Verification items for this drawing (mm, ordinates from the low corner). A direction names the side the tool comes from. Round coordinates to 2 decimals unless told otherwise and drop trailing zeros. Loops run counter-clockwise (first coordinate to the right, second up) from the corner with the lowest first, then second, coordinate; pieces in that order, holes last. Notation, with made-up numbers: M 35.25,-14.5 L 77.25,-14.5 A24 cw 77.25,-2.5 Z; hole C 79.25,-14.5 d6. An arc over 180 degrees is marked long. Write item = value, one per line. Start each with the question number.
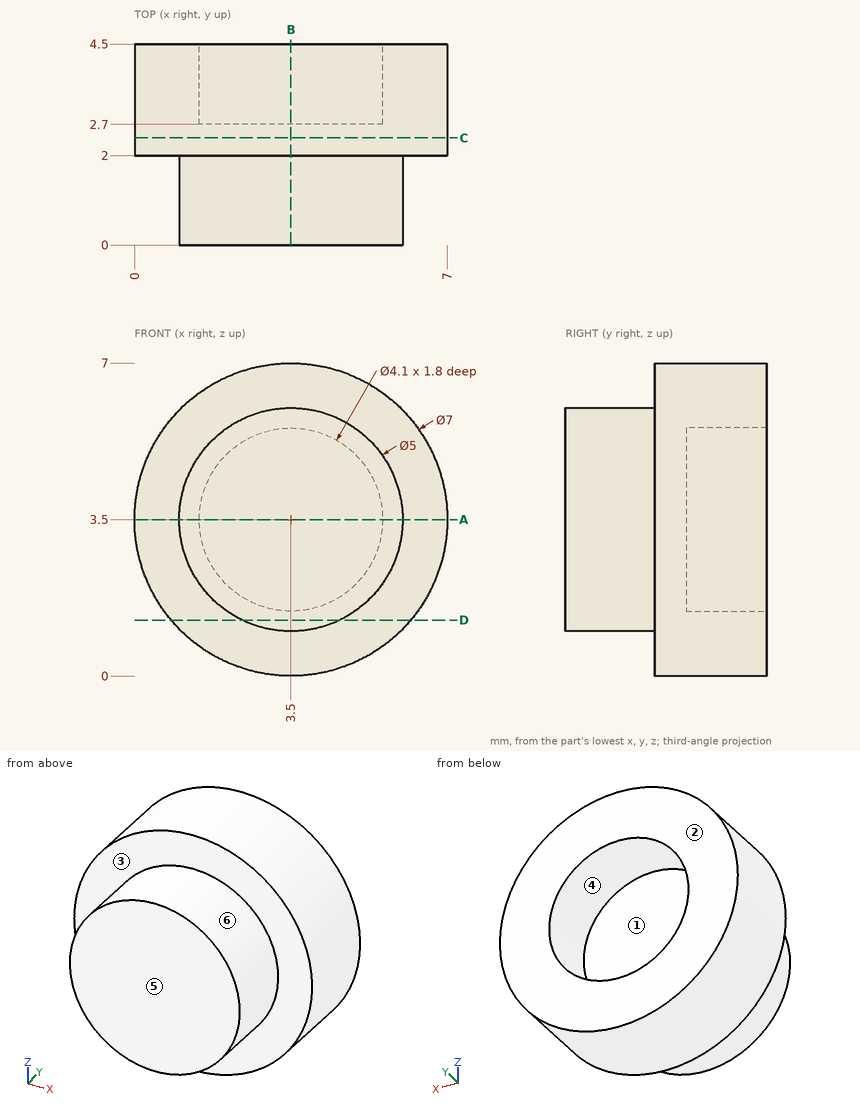
1. Section check D-D, the plane z = 1.25. Enter the section's corners in (x, y), and give its area (3 significant figures).
2. Section check C-C, the plane y = 2.4. Enter the section's corners in (x, z), and give its area (3 significant figures).
3. Thickness scan on line 1 (X direction, y = 3.7, z = 3.5); line 2 (Z direction, x = 4.5, y = 3.3); line 3 (Y direction, x = 6.5, z = 4.25). Record the ranges inside material, lowest first.
4. Tool access check on the marked faces 1, 2 and 3. Record the directions out of +Z, -Z, +X, -X, +Y, -Y that give a thin tool (end or side, any length) a straight path to the whole face; none if there is none.
5. Mould release check, pull along X, two halves, no side actions. Record for the marked faces 4, 5 and 6: pulls with the +X half, pulls with the -X half, needs draft (parallel to the pull), parting line crosses it, or undercut.
6. Section check B-B, the plane x = 3.5. Enter the section's corners in (y, z).
7. Section check A-A, the plane z = 3.5. Enter the section's corners in (x, y), and give its area (3 significant figures).
Computed values:
q1.outline = M 0.82,2 L 2.41,2 L 2.41,0 L 4.59,0 L 4.59,2 L 6.18,2 L 6.18,4.5 L 0.82,4.5 Z
q1.area = 17.8 mm2
q2.outline = C 3.5,3.5 d7
q2.area = 38.5 mm2
q3.line_1 = 0 to 1.45, 5.55 to 7
q3.line_2 = 0.15 to 1.71, 5.29 to 6.85
q3.line_3 = 2 to 4.5
q4.face_1 = +Y
q4.face_2 = +Z, -Z, +X, -X, +Y
q4.face_3 = -Y
q5.face_4 = undercut
q5.face_5 = needs draft
q5.face_6 = parting line crosses it
q6.outline = M 0,1 L 2,1 L 2,0 L 4.5,0 L 4.5,1.45 L 2.7,1.45 L 2.7,5.55 L 4.5,5.55 L 4.5,7 L 2,7 L 2,6 L 0,6 Z
q7.outline = M 0,2 L 1,2 L 1,0 L 6,0 L 6,2 L 7,2 L 7,4.5 L 5.55,4.5 L 5.55,2.7 L 1.45,2.7 L 1.45,4.5 L 0,4.5 Z
q7.area = 20.1 mm2
